```python
from build123d import *

# Parameters (mm, degrees)
SKETCH_1_R      = 1.5
EXTRUDE_1_DEPTH = 2
EXTRUDE_START   = 2
SKETCH_2_R      = 3.25
EXTRUDE_2_DEPTH = 1.5
SKETCH_3_R      = 4.5
EXTRUDE_3_DEPTH = 1


with BuildPart() as part:
    # 草图1 → 凸台-拉伸1 (new body)
    with BuildSketch(Plane(origin=(0, 0, 0), x_dir=(1, 0, 0), z_dir=(0, 1, 0))):
        with Locations(Location((0, 0, 0), (0, 0, 270))):
            Circle(SKETCH_1_R)
    extrude(amount=EXTRUDE_1_DEPTH)

    # 草图2 → 凸台-拉伸2 (add)
    with BuildSketch(Plane(origin=(0, 0, 0), x_dir=(1, 0, 0), z_dir=(0, 1, 0)).offset(EXTRUDE_START)):
        with Locations(Location((0, 0, 0), (0, 0, 270))):
            Circle(SKETCH_2_R)
    extrude(amount=EXTRUDE_2_DEPTH)

    # 草图3 → 凸台-拉伸3 (add)
    with BuildSketch(Plane(origin=(0, 0, 0), x_dir=(1, 0, 0), z_dir=(0, 1, 0))):
        with Locations(Location((0, 0, 0), (0, 0, 270))):
            Circle(SKETCH_3_R)
    extrude(amount=-EXTRUDE_3_DEPTH)

    # 草图4 → 旋转1 (revolve)
    with BuildSketch(Plane.XY):
        Polygon((4.5, -1), (10, -4.175426481), (8.5, -4.175426481), (3, -1), align=None)
    revolve(axis=Axis((0, -1000, 0), (0, 1, 0)))


solid = part.part
```
The model under review builds one solid part; all positions refer to its coordinate system, in mm. A direction names the side the tool comes from. Round coordinates to 2 decimals unless told otherwise and drop trailing zeros. Write each loop counter-clockwise with the first axis right and the second up, starting at its lowest first coordinate (ties: lowest second). Pieces come first, ordered by that corner, then holes. Notation, with made-up numbers: (2, 21.25) - (28, 21.25) arc R16 ccw to (28, 38.25) - close; hole circle Ø10 at (20, 82.25). An arc over 180 degrees is marked (long way). Answer as CSV lines item,"result". Start each with the question number.
(1) We need section C-C on y = 1.75. State the section outline as (x, z) points.
(2) We need section D-D on y = -2.75. State the section outline as (x, z) points, plus the area to 3 significant figures.
(3) Draft analysis for pull direction Z (two halves, no side actions). For faces 1 (the conical face through (-0.708, -1.154, 3.189)), 2 (the cylindrical face through (-1.978, 2.74, -2.579)), 3 (the flat face through (-4.5, -4.175, 7.4)), state which applies: pulls with the +Z half, pulls with the -Z half, needs draft (parallel to the pull), parting line crosses it, or undercut.
(4) We need section A-A on x = 0. State the section outline as (y, z) points, plus the area to 3 significant figures.
(5) For pin 1 Ø1.5 at (x, y) = (-1.5, 1.5) entering from +Z; pin 2 Ø1 at (x, z) = (-2.5, -4.5) entering from +Y; pin 3 Ø4 at (y, z) = (-1.5, 2) entering from +X; pin 4 Ø1.5 at (y, z) = (1, 6) entering from +X, all flat-tipped, find the tip position at first contact; note any pin that passes through.
(6) For faces 4 (the flat face through (0, -1, 0)), 5 (the cylindrical face through (1.352, -0.493, 4.292)), 6 (the cylindrical face through (0.45, 0.99, 1.43)), list the 3-axis set-ups (+Z, -Z, +X, -X, +Y, -Y) from which the entire face can be reached by the end or side of a thin tool; tool diameter is ignored.
(7) To check wall thickness, follow line 1 (Y direction, x = -1.25, z = 1.75); line 2 (X direction, y = -3.25, z = -4.5); line 3 (X direction, y = -3, z = 0.75). State the ranges of each line that lie inside material, in increasing order.
(8) We need section B-B on z = 0. State the section outline as (x, y) points, plus the area to 3 significant figures.
Worked answers:
1,outline,"circle Ø3 at (0, 0)"
2,outline,"circle Ø15.06 at (0, 0); hole circle Ø12.06 at (0, 0)"
2,area,"63.9 mm²"
3,face 1,"undercut"
3,face 2,"parting line crosses it"
3,face 3,"needs draft"
4,outline,"(-4.18, -10) - (-1, -4.5) - (0, -4.5) - (0, -1.5) - (2, -1.5) - (2, -3.25) - (3.5, -3.25) - (3.5, 3.25) - (2, 3.25) - (2, 1.5) - (0, 1.5) - (0, 4.5) - (-1, 4.5) - (-4.18, 10) - (-4.18, 8.5) - (-1, 3) - (-1, -3) - (-4.18, -8.5) - close"
4,area,"34.3 mm²"
5,pin 1,"z = 3.11"
5,pin 2,"y = -1.09"
5,pin 3,"x = 8.63"
5,pin 4,"through"
6,face 4,"-Y"
6,face 5,"+Y"
6,face 6,"none"
7,line 1,"-1 to 0, 2 to 3.5"
7,line 2,"-7.09 to -5.23, 5.23 to 7.09"
7,line 3,"-7.93 to -6.42, 6.42 to 7.93"
8,outline,"(-10, -4.18) - (-8.5, -4.18) - (-3, -1) - (3, -1) - (8.5, -4.18) - (10, -4.18) - (4.5, -1) - (4.5, 0) - (1.5, 0) - (1.5, 2) - (3.25, 2) - (3.25, 3.5) - (-3.25, 3.5) - (-3.25, 2) - (-1.5, 2) - (-1.5, 0) - (-4.5, 0) - (-4.5, -1) - close"
8,area,"34.3 mm²"
